from build123d import *

# Parameters (mm, degrees)
BOSS_EXTRUDE1_DEPTH = 1930
FILLET1_R           = 3
CUT_EXTRUDE1_DEPTH  = 88
CUT_EXTRUDE2_DEPTH  = 88


with BuildPart() as part:
    # Sketch1 → Boss-Extrude1 (new body)
    with BuildSketch(Plane(origin=(0, 0, 0), x_dir=(0, 0, -1), z_dir=(1, 0, 0))):
        Polygon((0, 0), (88, 0), (88, -88), (85, -88), (85, -3), (0, -3), align=None)
    extrude(amount=BOSS_EXTRUDE1_DEPTH)

    # Fillet1
    fillet1_edges = [part.edges().sort_by_distance(p)[0] for p in [
        (965, 0, -88),
        (965, -3, -85),
    ]]
    fillet(fillet1_edges, radius=FILLET1_R)

    # Sketch2 → Cut-Extrude1 (cut)
    with BuildSketch(Plane(origin=(0, 0, -88), x_dir=(-1, 0, 0), z_dir=(0, 0, -1))):
        Polygon((0, 0), (-88, -88), (0, -88), align=None)
    extrude(amount=-CUT_EXTRUDE1_DEPTH, mode=Mode.SUBTRACT)

    # Sketch3 → Cut-Extrude2 (cut)
    with BuildSketch(Plane(origin=(0, 0, -88), x_dir=(-1, 0, 0), z_dir=(0, 0, -1))):
        Polygon((-1930, 0), (-1842, -88), (-1930, -88), align=None)
    extrude(amount=-CUT_EXTRUDE2_DEPTH, mode=Mode.SUBTRACT)


solid = part.part
Input: part model. Units: mm. Frame: model coordinates. A direction names the side the tool comes from. Round coordinates to 2 decimals unless told otherwise and drop trailing zeros. Loops run counter-clockwise (first coordinate to the right, second up) from the corner with the lowest first, then second, coordinate; pieces in that order, holes last. Notation, with made-up numbers: M 45,75 L 51,75 A33 cw 51,110 Z; hole C -32,35.5 d5. An arc over 180 degrees is marked long. Answer as CSV lines item,"result". Start each with the question number.
(1) Line query: line 1 (Z direction, x = 242, y = -22.5); line 2 (Y direction, x = 573.5, z = -13.5). Output: solid intervals per line, ascending. Write a range as [from, to].
(2) Section A-A, the plane x = 713. Output: boundary loops of the cut face in (y, z).
(3) First-contact query: pin 1 (1 mm diameter, centred on x = 718.5, z = -10, fed in from -Y); pin 2 (8 mm diameter, centred on x = 377.5, y = -57, fed in from +Z). Flat tips, straight axial feed; report the tip coordinate or a pass-through.
(4) Section B-B, the plane y = -29.5. Output: boundary loops of the cut face in (x, z).
(5) Reachability of faces 1 (the flat face through (952, -3, -42)), 2 (the flat face through (1906, -24, -87)) from +Z, -Z, +X, -X, +Y, -Y: full face, straight path, thin tool, end or side. Return the list, or none.
(6) Section C-C, the plane z = -24.5. Output: boundary loops of the cut face in (x, y).
Values found:
1,line 1,"z = [-88, -85]"
1,line 2,"y = [-3, 0]"
2,outline,"M -88,-88 L -3,-88 A3 ccw 0,-85 L 0,0 L -3,0 L -3,-82 A3 cw -6,-85 L -88,-85 Z"
3,pin 1,"stops at y = -3"
3,pin 2,"stops at z = -85"
4,outline,"M 29.5,-88 L 1900.5,-88 L 1900.5,-85 L 29.5,-85 Z"
5,face 1,"+Z, +X, -X, -Y"
5,face 2,"+Z, -Z, +X, -Y"
6,outline,"M 0,0 L 3,-3 L 1927,-3 L 1930,0 Z"
